```python
from build123d import *

# Parameters (mm, degrees)
SKETCH_1_R               = 21
EXTRUDE_1_DEPTH          = 6
SKETCH_2_R               = 8
CUT_EXTRUDE_1_DEPTH      = 8
PATTERN_CIRCULAR_1_COUNT = 8
PATTERN_CIRCULAR_2_COUNT = 10


with BuildPart() as part:
    # Sketch 1 → Extrude 1 (new body)
    with BuildSketch(Plane.XY):
        Circle(SKETCH_1_R)
    extrude(amount=EXTRUDE_1_DEPTH)

    # Sketch 2 → Cut-Extrude 1 (cut)
    with BuildSketch(Plane(origin=(0, 0, 0), x_dir=(-1, 0, 0), z_dir=(0, 0, -1))):
        Circle(SKETCH_2_R)
    extrude(amount=-CUT_EXTRUDE_1_DEPTH, mode=Mode.SUBTRACT)

    # Sketch 7 → Hole Wizard 1 (revolve, cut)
    with BuildSketch(Plane(origin=(0, 11.25, 0), x_dir=(0, 1, 0), z_dir=(1, 0, 0))):
        Polygon((0, 0), (0, 8.581549114), (1.8, 7.5), (1.8, 3.4), (3, 3.4), (3, 0), align=None)
    hole_wizard_1 = revolve(axis=Axis((0, 11.25, -6.35), (0, 0, 1)), mode=Mode.SUBTRACT)

    # Pattern Circular 1: Hole Wizard 1 ×8 about axis
    pattern_circular_1_axis = Axis((0, 0, 0), (0, 0, 1))
    for i in range(1, PATTERN_CIRCULAR_1_COUNT):
        add(hole_wizard_1.rotate(pattern_circular_1_axis, i * 360 / PATTERN_CIRCULAR_1_COUNT), mode=Mode.SUBTRACT)

    # Sketch 13 → Hole Wizard 7 (revolve, cut)
    with BuildSketch(Plane(origin=(0, 17.5, 0), x_dir=(0, 1, 0), z_dir=(1, 0, 0))):
        Polygon((0, 0), (0, 8.581549114), (1.8, 7.5), (1.8, 3.4), (3, 3.4), (3, 0), align=None)
    hole_wizard_7 = revolve(axis=Axis((0, 17.5, -6.35), (0, 0, 1)), mode=Mode.SUBTRACT)

    # Pattern Circular 2: Hole Wizard 7 ×10 about axis
    pattern_circular_2_axis = Axis((0, 0, 0), (0, 0, 1))
    for i in range(1, PATTERN_CIRCULAR_2_COUNT):
        add(hole_wizard_7.rotate(pattern_circular_2_axis, i * 360 / PATTERN_CIRCULAR_2_COUNT), mode=Mode.SUBTRACT)


solid = part.part
```
Design review of the part built by this model. Coordinates are the model's own, in mm. A direction names the side the tool comes from. Coordinates: 2 decimals unless noted, no trailing zeros. Order: outer loops, then holes, each group sorted by start corner. A loop starts at its lowest first (then second) coordinate and runs counter-clockwise, first axis right, second up.
1) Take a section at B-B, the plane z = 1.85. State how many separate pieces and enclosed holes the cut face has, and give its area (3 significant figures).
2) For faces 1 (the cylindrical face through (12.845, 15.724, 1.676)), 2 (the cylindrical face through (-6.527, -9.051, 4.682)), list the 3-axis set-ups (+Z, -Z, +X, -X, +Y, -Y) from which the entire face can be reached by the end or side of a thin tool; tool diameter is ignored.
3) Wall thickness on line 1 along Y through (x, z) = (6.5, 2.9); line 2 along X through (y, z) = (-15.5, 1.05); line 3 along Y through (x, z) = (-13, 0.95): over which ranges is each line inside the solid? List them lowest first.
4) Take a section at A-A, the plane y = 0. Give the boundary of the cut face in (x, z), and give its area (3 significant figures).
5) Mouldability with a two-part tool opening along Y and no side actions: class faces 3 (the cylindrical face through (1.8, 15.1, 1.7)), 4 (the cylindrical face through (-0.08, 9.45, 4.68)) as +Y half, -Y half, draft (parallel to the pull), parting line (faces both ways), or undercut.
6) Clearance check with a flat-ended pin moving along its axis: pin 1 (1.5 mm diameter, centred on y = -1, z = 3, fed in from -X). State where the tip first meets the part, or that it passes through.
Returned:
1. separate pieces: 1
1. enclosed holes: 19
1. area: 675 mm2
2. face 1: -Z
2. face 2: +Z, -Z
3. line 1: y = -19.97 to -10.58, -5.33 to -4.66, 4.66 to 5.33, 10.58 to 19.97
3. line 2: x = -14.17 to -12.97, -7.6 to -2.24, 2.24 to 7.6, 12.97 to 14.17
3. line 3: y = -16.49 to -15.44, -12.88 to -2.44, 2.44 to 12.88, 15.44 to 16.49
4. outline: (-21, 0) - (-14.25, 0) - (-14.25, 3.4) - (-13.05, 3.4) - (-13.05, 6) - (-21, 6) - close; (-9.45, 3.4) - (-8.25, 3.4) - (-8.25, 0) - (-8, 0) - (-8, 6) - (-9.45, 6) - close; (8, 0) - (8.25, 0) - (8.25, 3.4) - (9.45, 3.4) - (9.45, 6) - (8, 6) - close; (13.05, 3.4) - (14.25, 3.4) - (14.25, 0) - (21, 0) - (21, 6) - (13.05, 6) - close
4. area: 96.5 mm2
5. face 3: undercut
5. face 4: undercut
6. pin 1: stops at x = -21
